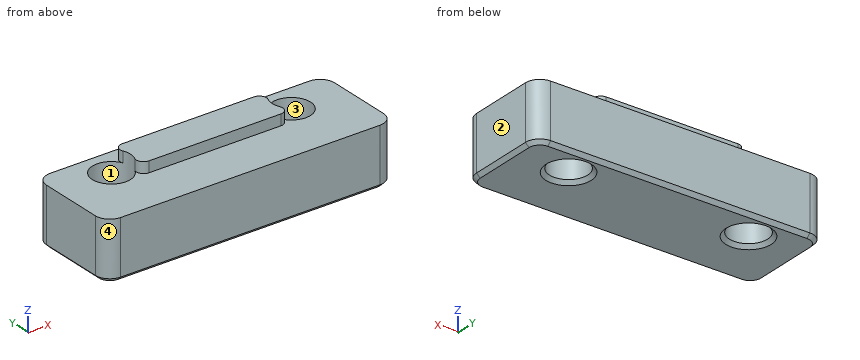
Autodesk Inventor part; units mm, degrees
ref_plane "YZ Plane" through (0, 0, 0) normal (1, 0, 0) x (0, 1, 0)
ref_plane "XZ Plane" through (0, 0, 0) normal (0, 1, 0) x (-1, 0, 0)
ref_plane "XY Plane" through (0, 0, 0) normal (0, 0, 1) x (1, 0, 0)
sketch "Sketch1" plane through (0, 0, 0) normal (0, 0, 1) x (1, 0, 0)
  line L0 (-20, -4) -> (20, -4)
  line L1 (20, -4) -> (20, 4)
  line L2 (20, 4) -> (-20, 4)
  line L3 (-20, 4) -> (-20, -4)
  line L4 (-20, -4) -> (20, 4) construction
  line L5 (20, -4) -> (-20, 4) construction
  point P0 (0, 0)
  dimension "d0" = 8
  dimension "d1" = 40
extrude "Extrusion1" add sketch "Sketch1" along normal blind 8
sketch "Sketch2" plane through (-20, -4, 0) normal (0, -1, 0) x (1, 0, 0)
  line L0 (0, 0) -> (40, 0)
  line L1 (40, 0) -> (40, 8)
  line L2 (0, 8) -> (40, 8)
  line L3 (0, 0) -> (0, 8)
  point P0 (20, 0)
extrude "Extrusion2" add sketch "Sketch2" along normal blind 5
sketch "Sketch3" plane through (0, 0, 8) normal (0, 0, 1) x (1, 0, 0)
  line L0 (-15, -3) -> (15, -3) construction
  line L1 (15, -3) -> (15, 3) construction
  line L2 (15, 3) -> (-15, 3) construction
  line L3 (-15, 3) -> (-15, -3) construction
  line L4 (-15, -3) -> (15, 3) construction
  line L5 (15, -3) -> (-15, 3) construction
  line L6 (-28, 0) -> (28, 0) construction
  circle A0 centre (-12.5, 0) radius 2.65
  line L7 (0, 6.6) -> (0, -11.6) construction
  line L8 (15, 3) -> (15, -3) construction
  circle A1 centre (12.5, 0) radius 2.65
  point P0 (0, 0)
  dimension "d6" = 6
  dimension "d7" = 30
  dimension "d8" = 5.3
  dimension "d20" = 25
extrude "Extrusion3" cut sketch "Sketch3" against normal through all
sketch "Sketch4" plane through (0, 0, 8) normal (0, 0, 1) x (1, 0, 0)
  line L0 (-13, -2.5) -> (13, -2.5)
  line L1 (13, -2.5) -> (13, 2.5)
  line L2 (13, 2.5) -> (-13, 2.5)
  line L3 (-13, 2.5) -> (-13, -2.5)
  line L4 (-13, -2.5) -> (13, 2.5) construction
  line L5 (13, -2.5) -> (-13, 2.5) construction
  circle A0 centre (-12.5, 0) radius 2.65
  circle A1 centre (12.5, 0) radius 2.65
  point P0 (0, 0)
  point P1 (-8.1211, 2.5)
  point P2 (-8.1211, -2.5)
  point P3 (-11.6211, -2.5)
  point P4 (-11.6211, 2.5)
  point P5 (11.6211, -2.5)
  point P6 (11.6211, 2.5)
  dimension "d11" = 26
  dimension "d12" = 5
extrude "Extrusion4" add sketch "Sketch4" along normal blind 1.5 contours A0 L2 A1 L0
fillet "Fillet1" radius 1 4 edges at (-11.6211, -2.5, 8.75) (-11.6211, 2.5, 8.75) (11.6211, -2.5, 8.75) (11.6211, 2.5, 8.75)
fillet "Fillet2" radius 2 4 edges at (-20, -9, 4) (-20, 4, 4) (20, -9, 4) (20, 4, 4)
chamfer "Chamfer1" distance 0.5 angle 45 6 edges at (0, -9, 0) (20, -2.5, 0) (0, 4, 0) (-20, -2.5, 0) (-15.15, 0, 0) (9.85, 0, 0)
properties part number "_3DPrint"
Source: CAD feature listing. Evaluate the final solid. Frame: model axes, mm. Face numbers are marked on the shaded views. Coordinates: 2 decimals unless noted, no trailing zeros. Write each loop counter-clockwise with the first axis right and the second up, starting at its lowest first coordinate (ties: lowest second). Pieces come first, ordered by that corner, then holes. Notation, with made-up numbers: M 53.25,29 L 94.25,29 A19 cw 94.25,57 Z; hole C 39.25,57 d10. An arc over 180 degrees is marked long. Answer as a JSON object with one key per item and string values.
1. Cut plane B-B on y = 0. Output: boundary loops of the cut face in (x, z), plus the area to 3 significant figures.
Evaluation:
{"outline": "M -20,0.5 L -19.5,0 L -15.65,0 L -15.15,0.5 L -15.15,8 L -20,8 Z; M -9.85,0.5 L -9.35,0 L 9.35,0 L 9.85,0.5 L 9.85,9.5 L -9.85,9.5 Z; M 15.15,0.5 L 15.65,0 L 19.5,0 L 20,0.5 L 20,8 L 15.15,8 Z", "area": "264 mm^2"}
2. Ray query, L1, parallel to X at y = 1.5, z = 4.75; L2, parallel to Y at x = -12.5, z = 6.5; L3, parallel to X at y = -1.25, z = 2.5. Return the intervals inside material, ascending.
Evaluation:
{"L1": "-20 to -14.68, -10.32 to 10.32, 14.68 to 20", "L2": "-9 to -2.65, 2.65 to 4", "L3": "-20 to -14.84, -10.16 to 10.16, 14.84 to 20"}
3. Draft query along Y for the marked faces 1, 2, 3 and 4. Return one class per face: released by +Y, released by -Y, zero draft, split by the parting line, or undercut.
Evaluation:
{"face 1": "undercut", "face 2": "zero draft", "face 3": "undercut", "face 4": "released by -Y"}
4. Cut plane C-C on x = 12.5. Output: boundary loops of the cut face in (y, z).
Evaluation:
{"outline": "M -9,0.5 L -8.5,0 L -3.15,0 L -2.65,0.5 L -2.65,8 L -9,8 Z; M 2.65,0.5 L 3.15,0 L 3.5,0 L 4,0.5 L 4,8 L 2.65,8 Z"}
5. Cut plane A-A on z = 6. Output: boundary loops of the cut face in (x, y).
Evaluation:
{"outline": "M -20,-7 A2 ccw -18,-9 L 18,-9 A2 ccw 20,-7 L 20,2 A2 ccw 18,4 L -18,4 A2 ccw -20,2 Z; hole C -12.5,0 d5.3; hole C 12.5,0 d5.3"}
6. Cut plane D-D on x = -2. Output: boundary loops of the cut face in (y, z).
Evaluation:
{"outline": "M -9,0.5 L -8.5,0 L 3.5,0 L 4,0.5 L 4,8 L 2.5,8 L 2.5,9.5 L -2.5,9.5 L -2.5,8 L -9,8 Z"}
7. Contact query for flat-ended pins moving along their axis: P1, Ø1.2, axis at x = -3.5, z = 8.5, coming from the +Y side; P2, Ø5, axis at x = 12.5, y = 0, coming from the +Z side; P3, Ø3, axis at x = -14, y = -2.5, coming from the +Z side. Output: stop coordinate, or through.
Evaluation:
{"P1": "y = 4", "P2": "through", "P3": "z = 8"}
